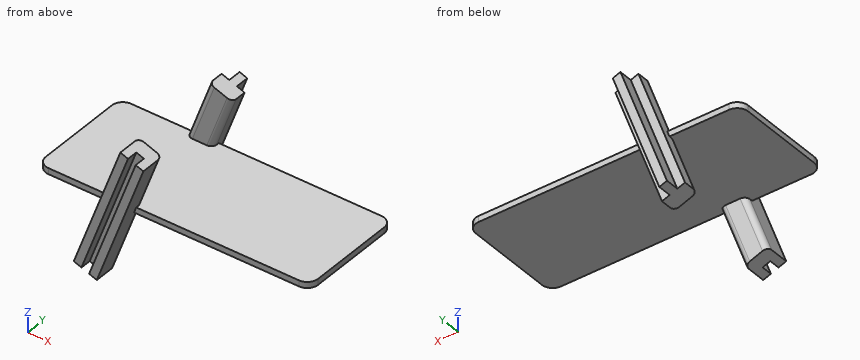
from build123d import *

# Parameters (mm, degrees)
F0_W          = 30.6458014898
F0_H          = 40
F0_W_2        = 69.3541985102
F1_DEPTH      = 2.2
F4_DEPTH      = 25
F4_DEPTH_BACK = 25
F5_R          = 4
F6_R          = 2


# Not quite as in the source:
# - a feature names something its author has since deleted; it is built from what else it names


with BuildPart() as f1:
    # F0 (on Top) → F1 (new body)
    with BuildSketch(Plane.XY):
        with Locations((-27.8972219743, -2.6114098728)):
            Rectangle(F0_W, F0_H)
        with Locations((22.1027780257, -2.6114098728)):
            Rectangle(F0_W_2, F0_H)
    extrude(amount=F1_DEPTH)

    # F3 (on line) → F4 (join, two sides)
    with BuildSketch(Plane(origin=(-1.4709161628, 0, -4.0413089432), x_dir=(0.9396926208, 0, -0.3420201433), z_dir=(-0.3420201433, 0, -0.9396926208))) as f4_sk:
        Polygon((-7.3159968707, -20.3885901272), (-7.3159968707, -14.3885901272), (-11.8159968707, -14.3885901272), (-11.8159968707, -25.3885901272), (-10.3159968707, -25.3885901272), (-10.3159968707, -20.3885901272), align=None)
        Polygon((-11.8159968707, 19.6114098728), (-7.3159968707, 19.6114098728), (-7.3159968707, 28.6114098728), (-10.3159968707, 28.6114098728), (-10.3159968707, 24.6114098728), (-11.8159968707, 24.6114098728), align=None)
        Polygon((-11.8159968707, -25.3885901272), (-11.8159968707, -14.3885901272), (-16.3159968707, -14.3885901272), (-16.3159968707, -20.3885901272), (-13.3159968707, -20.3885901272), (-13.3159968707, -25.3885901272), align=None)
        Polygon((-16.3159968707, 19.6114098728), (-11.8159968707, 19.6114098728), (-11.8159968707, 24.6114098728), (-13.3159968707, 24.6114098728), (-13.3159968707, 28.6114098728), (-16.3159968707, 28.6114098728), align=None)
    extrude(amount=F4_DEPTH)
    extrude(f4_sk.sketch, amount=-F4_DEPTH_BACK)

    # F5
    f5_edges = [f1.edges().sort_by_distance(p)[0] for p in [
        (-43.220123, 17.38859, 1.1),
        (-43.220123, -22.61141, 1.1),
        (56.779877, -22.61141, 1.1),
        (56.779877, 17.38859, 1.1),
    ]]
    fillet(f5_edges, radius=F5_R)

    # F6
    f6_edges = [f1.edges().sort_by_distance(p)[0] for p in [
        (-3.389994, -19.61141, 12.076612),
        (-12.407411, -19.61141, 13.615703),
        (-3.389994, 14.38859, 12.076612),
        (-12.340865, 14.38859, -12.515703),
        (-12.407411, 14.38859, 13.615703),
        (-21.358281, 14.38859, -10.976612),
        (-21.358281, -19.61141, -10.976612),
        (-12.340865, -19.61141, -12.515703),
    ]]
    fillet(f6_edges, radius=F6_R)


solid = f1.part
Build history of the part. All positions in model axes, mm. Round coordinates to 2 decimals unless told otherwise and drop trailing zeros. Write each loop counter-clockwise with the first axis right and the second up, starting at its lowest first coordinate (ties: lowest second). Pieces come first, ordered by that corner, then holes. Notation, with made-up numbers: M 38.5,83 L 68.5,83 A29 cw 68.5,110 Z; hole C 3.5,52.5 d6. An arc over 180 degrees is marked long. Answer in a Markdown table with one row per item.
1. Flat gauge pins, fed straight in: P1, Ø1.1, axis at x = -26, z = 1.5, coming from the +Y side; P2, Ø3, axis at x = -25, y = 5.5, coming from the +Z side; P3, Ø1.8, axis at x = 7.5, z = 1.5, coming from the -Y side. Where does each tip first touch, or does it go through?
Geometry check:
| item | result |
|---|---|
| P1 | y = 17.39 |
| P2 | z = 2.2 |
| P3 | y = -22.61 |
2. Probe L1, parallel to Z at x = -14.5, y = -8.5; L2, parallel to Y at x = 36.5, z = 2; L3, parallel to X at y = 17, z = 16. List the from-to ranges inside material, lowest first. Write a range as [from, to].
Geometry check:
| item | result |
|---|---|
| L1 | [0, 2.2] |
| L2 | [-22.61, 17.39] |
| L3 | [-11.54, -1.96] |
3. Saw through at A-A (y = -15). List the corners of the cut face in (x, z).
Geometry check:
| item | result |
|---|---|
| outline | M -43.22,0 L 56.78,0 L 56.78,2.2 L -43.22,2.2 Z |
4. Saw through at B-B (x = 21). List the corners of the cut face in (y, z), and give its area (3 significant figures).
Geometry check:
| item | result |
|---|---|
| outline | M -22.61,0 L 17.39,0 L 17.39,2.2 L -22.61,2.2 Z |
| area | 88.0 mm2 |
